Job drawing, mm, ordinate dimensions from the low corner. One solid piece. A direction names the side the tool comes from. Give positions to 0.01 mm unless a question says otherwise; leave off trailing zeros. Write each loop counter-clockwise with the first axis right and the second up, starting at its lowest first coordinate (ties: lowest second). Pieces come first, ordered by that corner, then holes. Notation, with made-up numbers: (-27.75, 67.5) - (26.25, 67.5) arc R13 cw to (26.25, 91.5) - close; hole circle Ø9 at (1.25, 48.5). An arc over 180 degrees is marked (long way). Answer as a JSON object with one key per item and string values.
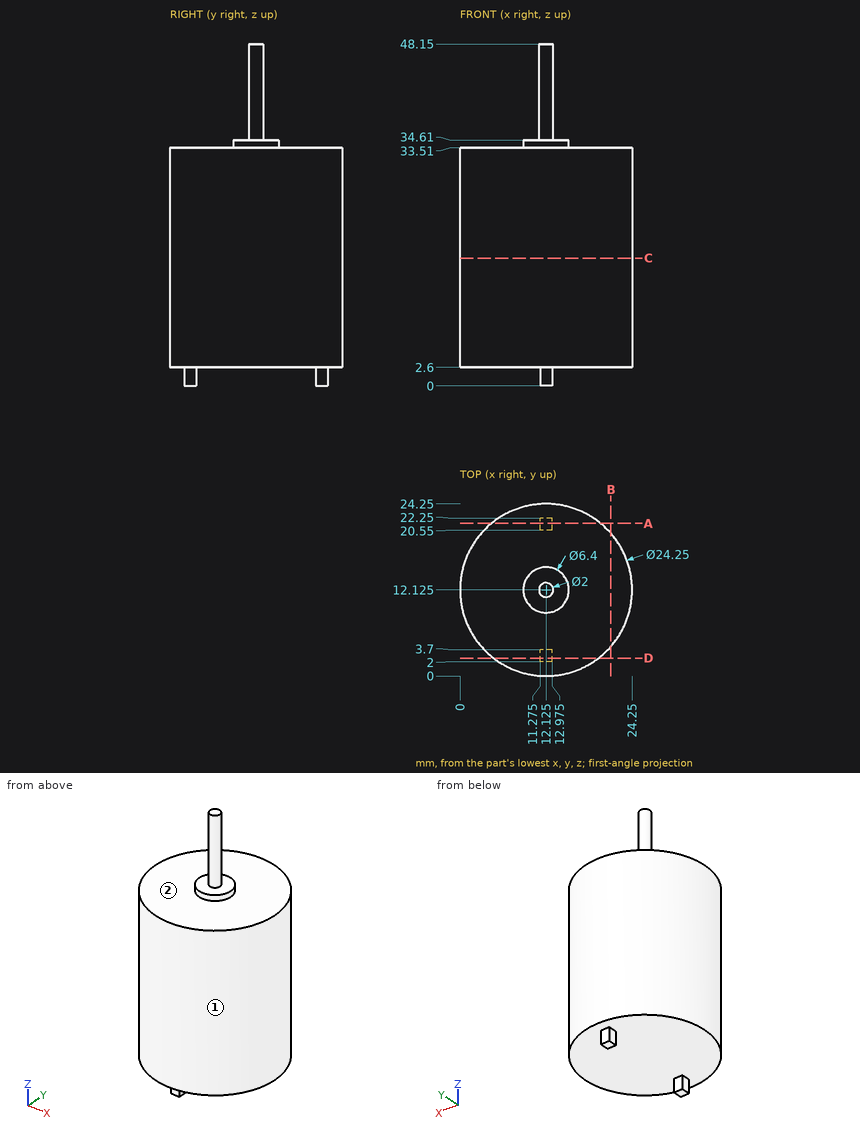
Item 1: Cut at C-C (z = 18). Give the cut face in (x, y) (3 decimals), and give its area (3 significant figures).
Entries:
{"outline": "circle Ø24.25 at (12.125, 12.125)", "area": "462 mm2"}
Item 2: Cut at B-B (x = 21.25). Give the cut face in (y, z), and give its area (3 significant figures).
Entries:
{"outline": "(4.14, 2.6) - (20.11, 2.6) - (20.11, 33.51) - (4.14, 33.51) - close", "area": "494 mm2"}
Item 3: Probe line 1 (Z direction, x = 13.5, y = 21.75); line 2 (Y direction, x = 11.25, z = 33); line 3 (X direction, y = 6, z = 18). List the from-to ranges inside material, lowest first. Write a range as from..to.
Entries:
{"line 1": "2.6..33.51", "line 2": "0.03..24.22", "line 3": "1.66..22.59"}
Item 4: Cut at A-A (y = 21.5). Give the cut face in (x, z) (3 decimals), and give its area (3 significant figures).
Entries:
{"outline": "(4.436, 2.6) - (11.275, 2.6) - (11.275, 0) - (12.975, 0) - (12.975, 2.6) - (19.814, 2.6) - (19.814, 33.51) - (4.436, 33.51) - close", "area": "480 mm2"}
Item 5: Which spindle directions (+Z, -Z, +X, -X, +Y, -Y) get a long thin tool onto all of the face, cutting with end or side? Do the marked faces 1 and 2. Say none if no direction does.
Entries:
{"face 1": "+Z, -Z", "face 2": "+Z"}
Item 6: Flat gauge pins, fed straight in: P1, Ø3, axis at x = 8.5, y = 3, coming from the -Z side; P2, Ø0.5, axis at x = 12, z = 1.5, coming from the -Y side; P3, Ø1.9, axis at x = 12, z = 1.5, coming from the +Y side. Where does each tip first touch, or does it go through?
Entries:
{"P1": "z = 2.6", "P2": "y = 2", "P3": "y = 22.25"}
Item 7: Cut at D-D (y = 2.5). Give the cut face in (x, z) (3 decimals), and give its area (3 significant figures).
Entries:
{"outline": "(4.751, 2.6) - (11.275, 2.6) - (11.275, 0) - (12.975, 0) - (12.975, 2.6) - (19.499, 2.6) - (19.499, 33.51) - (4.751, 33.51) - close", "area": "460 mm2"}
